```python
from build123d import *

# Parameters (mm, degrees)
BOSS_EXTRUDE1_DEPTH     = 45
CUT_EXTRUDE1_REACH      = 71.642
SKETCH2_R               = 12.5
CUT_EXTRUDE2_REACH      = 62.415
CUT_EXTRUDE2_END_RADIUS = 12.5
SKETCH3_R               = 5


with BuildPart() as part:
    # Sketch1 → Boss-Extrude1 (new, symmetric)
    with BuildSketch(Plane(origin=(0, 0, 0), x_dir=(0, 0, -1), z_dir=(1, 0, 0))):
        with BuildLine():
            Line((-20, 0), (20, 0))
            Line((20, 0), (20, 35))
            Line((20, 35), (12.5, 35))
            ThreePointArc((12.5, 35), (0, 22.5), (-12.5, 35))
            Line((-12.5, 35), (-20, 35))
            Line((-20, 35), (-20, 0))
        make_face()
    extrude(amount=BOSS_EXTRUDE1_DEPTH, both=True)

    # Sketch2 → Cut-Extrude1 (cut, up to next)
    with BuildSketch(Plane.XY.offset(20), mode=Mode.PRIVATE) as cut_extrude1_sk1:
        Circle(SKETCH2_R)
    cut_extrude1_tool1 = extrude(cut_extrude1_sk1.sketch, amount=-CUT_EXTRUDE1_REACH, mode=Mode.PRIVATE) & part.part
    add(cut_extrude1_tool1.solids().sort_by_distance((0, 0, 20))[0], mode=Mode.SUBTRACT)

    # Cut-Extrude2: up to this cylinder (the profile starts outside it)
    cut_extrude2_end = Plane(origin=(0, 35, 0), z_dir=(-1, 0, 0)) * Cylinder(CUT_EXTRUDE2_END_RADIUS, 214.83, mode=Mode.PRIVATE)
    # Sketch3 → Cut-Extrude2 (cut, up to the surface)
    with BuildSketch(Plane.XZ, mode=Mode.PRIVATE) as cut_extrude2_sk1:
        with Locations(Location((32, 0, 0), (0, 0, 270))):
            Circle(SKETCH3_R)
    cut_extrude2_tool1 = extrude(cut_extrude2_sk1.sketch, amount=-CUT_EXTRUDE2_REACH, mode=Mode.PRIVATE) - cut_extrude2_end
    add(cut_extrude2_tool1.solids().sort_by_distance((32, 0, 0))[0], mode=Mode.SUBTRACT)
    # Sketch3 → Cut-Extrude2 (cut, up to the surface)
    with BuildSketch(Plane.XZ, mode=Mode.PRIVATE) as cut_extrude2_sk2:
        with Locations(Location((-32, 0, 0), (0, 0, 270))):
            Circle(SKETCH3_R)
    cut_extrude2_tool2 = extrude(cut_extrude2_sk2.sketch, amount=-CUT_EXTRUDE2_REACH, mode=Mode.PRIVATE) - cut_extrude2_end
    add(cut_extrude2_tool2.solids().sort_by_distance((-32, 0, 0))[0], mode=Mode.SUBTRACT)


solid = part.part
```
Source: CAD feature listing. Evaluate the final solid. Frame: model axes, mm. Round coordinates to 2 decimals unless told otherwise and drop trailing zeros. Loops run counter-clockwise (first coordinate to the right, second up) from the corner with the lowest first, then second, coordinate; pieces in that order, holes last. Notation, with made-up numbers: M 80.25,63 L 99.25,63 A23 ccw 99.25,94 Z; hole C 31.5,53 d9. An arc over 180 degrees is marked long. Use a Markdown table: item, result. Add a question column.
1. Section query D-D on y = 17. Return the cut outline in (x, z).
2. Section query A-A on x = -32. Return the cut outline in (y, z), then the cut area to 3 significant figures.
3. Section query C-C on z = 0. Return the cut outline in (x, y).
4. Contact query for flat-ended pins moving along their axis: P1, Ø8, axis at x = 32, z = 0, coming from the -Y side; P2, Ø3, axis at x = 11, z = 5, coming from the +Y side; P3, Ø16, axis at x = -32, z = 0, coming from the +Y side; P4, Ø2, axis at x = 21.5, z = 4.5, coming from the -Y side. Output: stop coordinate, or through.
5. Section query B-B on y = 8.5. Return the cut outline in (x, z), then the cut area to 3 significant figures.
6. Line query: line 1 (X direction, y = 13.25, z = 0); line 2 (Z direction, x = 32, y = 9); line 3 (X direction, y = 13, z = 1). Output: solid intervals per line, ascending.
Reported:
| question | item | result |
|---|---|---|
| 1 | outline | M -45,-20 L 45,-20 L 45,20 L -45,20 Z; hole C -32,0 d10; hole C 32,0 d10 |
| 2 | outline | M 0,-20 L 35,-20 L 35,-12.5 A12.5 cw 23.54,-5 L 0,-5 Z; M 0,5 L 23.54,5 A12.5 cw 35,12.5 L 35,20 L 0,20 Z |
| 2 | area | 926 mm² |
| 3 | outline | M -45,0 L -37,0 L -37,22.5 L -45,22.5 Z; M -27,0 L -12.5,0 A12.5 cw 12.5,0 L 27,0 L 27,22.5 L -27,22.5 Z; M 37,0 L 45,0 L 45,22.5 L 37,22.5 Z |
| 4 | P1 | passes through |
| 4 | P2 | stops at y = 24.32 |
| 4 | P3 | stops at y = 25.4 |
| 4 | P4 | stops at y = 0 |
| 5 | outline | M -45,-20 L -9.17,-20 L -9.17,20 L -45,20 Z; M 9.17,-20 L 45,-20 L 45,20 L 9.17,20 Z; hole C -32,0 d10; hole C 32,0 d10 |
| 5 | area | 2,710 mm² |
| 6 | line 1 | x = -45 to -37, -27 to 27, 37 to 45 |
| 6 | line 2 | z = -20 to -5, 5 to 20 |
| 6 | line 3 | x = -45 to -36.9, -27.1 to 27.1, 36.9 to 45 |
